from build123d import *

# Parameters (mm, degrees)
F0_W     = 59.69
F0_H     = 59.69
F1_DEPTH = 25.4
F3_DEPTH = 10.16


with BuildPart() as f1:
    # F0 (on Top) → F1 (new body)
    with BuildSketch(Plane.XY):
        with Locations((40.005, 40.005)):
            Rectangle(F0_W, F0_H)
    extrude(amount=F1_DEPTH)



with BuildPart() as f1b:
    # F0 (on Top) → F1, piece 2 (new body)
    with BuildSketch(Plane.XY):
        with Locations((40.005, -40.005)):
            Rectangle(F0_W, F0_H)
    extrude(amount=F1_DEPTH)


with BuildPart() as f1c:
    # F0 (on Top) → F1, piece 3 (new body)
    with BuildSketch(Plane.XY):
        with Locations((-40.005, -40.005)):
            Rectangle(F0_W, F0_H)
    extrude(amount=F1_DEPTH)


with BuildPart() as f1d:
    # F0 (on Top) → F1, piece 4 (new body)
    with BuildSketch(Plane.XY):
        with Locations((-40.005, 40.005)):
            Rectangle(F0_W, F0_H)
    extrude(amount=F1_DEPTH)


with BuildPart() as f1_1:
    add(f1.part)

    add(f1b.part)  # F3 merges F1b

    add(f1c.part)  # F3 merges F1c

    add(f1d.part)  # F3 merges F1d
    # F2 (on Top) → F3 (join)
    with BuildSketch(Plane.XY):
        Polygon((10.16, 69.85), (-10.16, 69.85), (-10.16, 10.16), (-69.85, 10.16), (-69.85, -10.16), (-10.16, -10.16), (-10.16, -69.85), (10.16, -69.85), (10.16, -10.16), (69.85, -10.16), (69.85, 10.16), (10.16, 10.16), align=None)
    extrude(amount=F3_DEPTH)


solid = f1_1.part
CAD build for the part. Positions are in the model's coordinates, mm. A direction names the side the tool comes from. Round coordinates to 2 decimals unless told otherwise and drop trailing zeros. Order: outer loops, then holes, each group sorted by start corner. A loop starts at its lowest first (then second) coordinate and runs counter-clockwise, first axis right, second up. Notation, with made-up numbers: (-15.5, 74.5) -> (12.5, 74.5) arc R14 ccw to (12.5, 78.5) -> close; hole circle Ø6 at (64, 74). An arc over 180 degrees is marked (long way). Write each question's results on one line, items separated by ' | '.
1. Wall check: line 1 along X through (y, z) = (62, 23); line 2 along Z through (x, y) = (-4.5, -14.5). Give the ranges that are in metal, low to high. Write a range as [from, to].
Findings below:
line 1: x = [-69.85, -10.16], [10.16, 69.85] | line 2: z = [0, 10.16]
2. Cut at A-A (z = 14.75). Give the cut face in (x, y).
Findings below:
outline: (-69.85, -69.85) -> (-10.16, -69.85) -> (-10.16, -10.16) -> (-69.85, -10.16) -> close; (-69.85, 10.16) -> (-10.16, 10.16) -> (-10.16, 69.85) -> (-69.85, 69.85) -> close; (10.16, -69.85) -> (69.85, -69.85) -> (69.85, -10.16) -> (10.16, -10.16) -> close; (10.16, 10.16) -> (69.85, 10.16) -> (69.85, 69.85) -> (10.16, 69.85) -> close
3. Flat gauge pin, fed straight in: P1, Ø6, axis at x = 2, y = -33, coming from the +Z side. Where does the tip first touch, or does it go through?
Findings below:
P1: stops at z = 10.16
4. Cut at B-B (y = 22). Give the cut face in (x, z), plus the area to 3 significant figures.
Findings below:
outline: (-69.85, 0) -> (69.85, 0) -> (69.85, 25.4) -> (10.16, 25.4) -> (10.16, 10.16) -> (-10.16, 10.16) -> (-10.16, 25.4) -> (-69.85, 25.4) -> close | area: 3,240 mm²
5. 3-axis set-ups, long thin cutter, end or side, ignore diameter. For faces 5 (the face through (-40, -10.16, 18)), 6 (the face through (40, 40, 25.4)), 7 (the face through (10.16, 40, 18)): which of +Z, -Z, +X, -X, +Y, -Y reach the whole face in a straight line?
Findings below:
face 5: +Z, +X, -X | face 6: +Z, +X, -X, +Y, -Y | face 7: +Z, +Y, -Y
6. Cut at D-D (y = 3). Give the cut face in (x, z), plus the area to 3 significant figures.
Findings below:
outline: (-69.85, 0) -> (69.85, 0) -> (69.85, 10.16) -> (-69.85, 10.16) -> close | area: 1,420 mm²
7. Pull direction Y, two halves, no side cores. Call faces 1 (the face through (-1, -69.85, 10)), 2 (the face through (69.85, -1, 10)), 3 (the face through (0, -5, 10.16)), 4 (the face through (40, 10.16, 18)): pulls with the +Y half, pulls with the -Y half, needs draft (parallel to the pull), parting line crosses it, or undercut.
Findings below:
face 1: pulls with the -Y half | face 2: needs draft | face 3: undercut | face 4: undercut
